```python
from build123d import *

# Parameters (mm, degrees)
SKETCH2_R           = 1.5875
EXTRUDE1_DEPTH      = 12.7
EXTRUDE1_DEPTH_BACK = 12.7
CHAMFER1_SIZE       = 0.3175
SKETCH4_R           = 1.5875
SKETCH4_R_2         = 1.5621
CUT_EXTRUDE2_DEPTH  = 0.05
SKETCH5_R           = 1.5875
SKETCH5_R_2         = 1.5621
CUT_EXTRUDE3_DEPTH  = 0.05


with BuildPart() as part:
    # Sketch2 → Extrude1 (new body, two sides)
    with BuildSketch(Plane(origin=(0, 0, 0), x_dir=(0, 0, -1), z_dir=(1, 0, 0))) as extrude1_sk:
        Circle(SKETCH2_R)
    extrude(amount=EXTRUDE1_DEPTH)
    extrude(extrude1_sk.sketch, amount=-EXTRUDE1_DEPTH_BACK)

    # Chamfer1
    chamfer1_edges = [part.edges().sort_by_distance(p)[0] for p in [
        (-12.7, 0, 1.5875),
        (12.7, 0, 1.5875),
    ]]
    chamfer(chamfer1_edges, length=CHAMFER1_SIZE)

    # Sketch4 → Cut-Extrude2 (cut, symmetric)
    with BuildSketch(Plane.ZY.offset(6.35)):
        Circle(SKETCH4_R)
        Circle(SKETCH4_R_2, mode=Mode.SUBTRACT)
    extrude(amount=CUT_EXTRUDE2_DEPTH, both=True, mode=Mode.SUBTRACT)

    # Sketch5 → Cut-Extrude3 (cut, symmetric)
    with BuildSketch(Plane(origin=(6.35, 0, 0), x_dir=(0, 0, -1), z_dir=(1, 0, 0))):
        Circle(SKETCH5_R)
        Circle(SKETCH5_R_2, mode=Mode.SUBTRACT)
    extrude(amount=CUT_EXTRUDE3_DEPTH, both=True, mode=Mode.SUBTRACT)


solid = part.part
```
Could you check a few things on this model? Use its own coordinates, in mm. Give positions to 0.01 mm unless a question says otherwise; leave off trailing zeros. Write each loop counter-clockwise with the first axis right and the second up, starting at its lowest first coordinate (ties: lowest second). Pieces come first, ordered by that corner, then holes. Notation, with made-up numbers: (72, 19.5) -> (115, 19.5) arc R22 cw to (115, 56.5) -> close; hole circle Ø7 at (85.25, -13). An arc over 180 degrees is marked (long way). Write each question's results on one line, items separated by ' | '.
1. I need wall thicknesses on L1, parallel to Z at x = 3.5, y = 0.25; L2, parallel to X at y = 1.1, z = -0.7; L3, parallel to Y at x = 0.5, z = -0.1. Which ranges of each line are inside material? Lowest first, please.
Check sheet entries:
L1: z = -1.57 to 1.57 | L2: x = -12.67 to 12.67 | L3: y = -1.58 to 1.58
2. Will this pin go through, and if not, where does the flat tip stop? pin 1 Ø1 at (x, z) = (1, 0.5) entering from -Y.
Check sheet entries:
pin 1: stops at y = -1.59
3. I want a section at A-A, the plane x = 8.75. Write out the boundary of the cut face in (y, z) (1 decimal).
Check sheet entries:
outline: circle Ø3.2 at (0, 0)
